Check sheet for the modelled part. Datum: model origin and axes. Units: mm. Face numbers are marked on the shaded views. Coordinates: 2 decimals unless noted, no trailing zeros. Order: outer loops, then holes, each group sorted by start corner. A loop starts at its lowest first (then second) coordinate and runs counter-clockwise, first axis right, second up.
1. Gauge pin test, flat ends, axial feed: pin 1 Ø2 at (x, z) = (-2.5, -7.5) entering from -Y; pin 2 Ø1 at (x, y) = (-1, -5.5) entering from +Z; pin 3 Ø2 at (x, y) = (0.5, -0.5) entering from -Z. Record the tip position at first contact, or that the pin passes through.
2. Cross-section at D-D (x = 3.25). Enter the section's corners in (y, z).
3. Cross-section at B-B (y = 0). Enter the section's corners in (x, z), then the cut area to 3 significant figures.
4. Cross-section at C-C (y = 16). Enter the section's corners in (x, z).
5. Thickness scan on line 1 (Z direction, x = -1.25, y = 0); line 2 (Z direction, x = 2.75, y = 0); line 3 (Y direction, x = -2, z = 15). Record the ranges inside material, lowest first.
6. Cross-section at A-A (z = 0). Enter the section's corners in (x, y), then the cut area to 3 significant figures.
7. Draft check along Z on the marked faces 1, 2 and 3. Enter one of: released by +Z, released by -Z, zero draft, split by the parting line, or undercut.
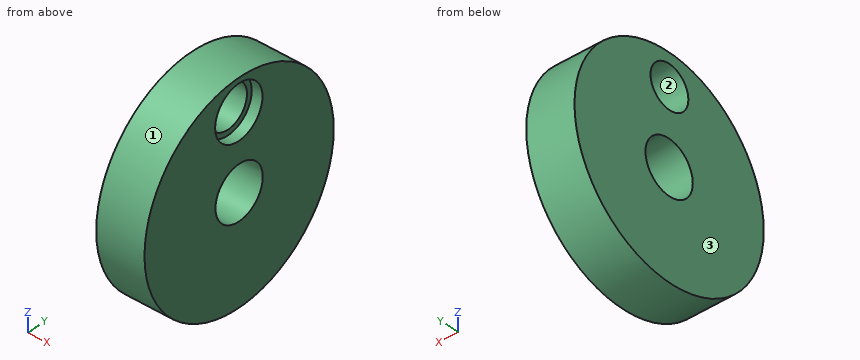
```python
from build123d import *

# Parameters (mm, degrees)
F0_R           = 20
F1_DEPTH       = 4.5
F3_D           = 10
F4_D           = 8
F4_CBORE_D     = 10
F4_CBORE_DEPTH = 2


with BuildPart() as f1:
    # F0 (on Right) → F1 (new body, symmetric)
    with BuildSketch(Plane.YZ):
        Circle(F0_R)
    extrude(amount=F1_DEPTH, both=True)

    # F3 (through all)
    with Locations(Plane.YZ.offset(4.5)):
        with Locations((0, 0)):
            Hole(F3_D / 2)

    # F4 (through all)
    with Locations(Plane.YZ.offset(4.5)):
        with Locations((-0.062594, 13.99986)):
            CounterBoreHole(F4_D / 2, F4_CBORE_D / 2, F4_CBORE_DEPTH)


solid = f1.part
```
Data:
1. pin 1: stops at y = -18.91
1. pin 2: stops at z = 19.36
1. pin 3: stops at z = -20
2. outline: circle Ø40 at (0, 0); hole circle Ø10 at (-0.06, 14); hole circle Ø10 at (0, 0)
3. outline: (-4.5, -20) - (4.5, -20) - (4.5, -5) - (-4.5, -5) - close; (-4.5, 5) - (4.5, 5) - (4.5, 9) - (2.5, 9) - (2.5, 10) - (-4.5, 10) - close; (-4.5, 18) - (2.5, 18) - (2.5, 19) - (4.5, 19) - (4.5, 20) - (-4.5, 20) - close
3. area: 194 mm2
4. outline: (-4.5, -12) - (4.5, -12) - (4.5, 12) - (-4.5, 12) - close
5. line 1: z = -20 to -5, 5 to 10, 18 to 20
5. line 2: z = -20 to -5, 5 to 9, 19 to 20
5. line 3: y = -13.23 to -3.94, 3.81 to 13.23
6. outline: (-4.5, -20) - (4.5, -20) - (4.5, -5) - (-4.5, -5) - close; (-4.5, 5) - (4.5, 5) - (4.5, 20) - (-4.5, 20) - close
6. area: 270 mm2
7. face 1: split by the parting line
7. face 2: undercut
7. face 3: zero draft
